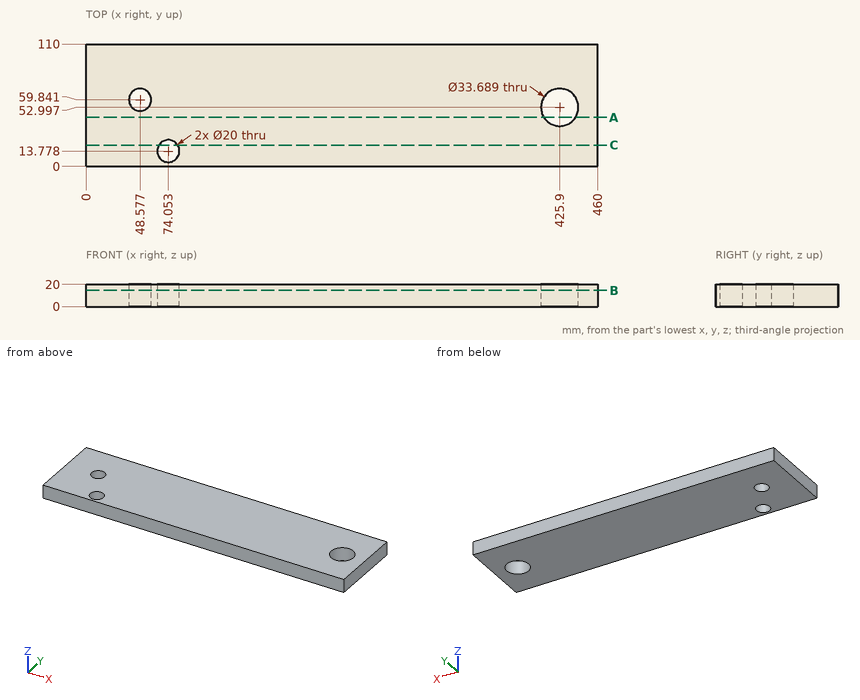
Design review of the part shown in the three views and the two pictorial views. Dimensions are in mm from the part's minimum x, y and z. Round coordinates to 2 decimals unless told otherwise and drop trailing zeros. Order: outer loops, then holes, each group sorted by start corner. A loop starts at its lowest first (then second) coordinate and runs counter-clockwise, first axis right, second up. Notation, with made-up numbers: (24, -4.5) -> (29, -4.5) arc R19 cw to (29, 24.5) -> close; hole circle Ø3 at (30.5, 6). An arc over 180 degrees is marked (long way). Write item = value, one per line. Start each with the question number.
1) Take a section at B-B on z = 14.5. State the section outline as (x, y) points (1 decimal).
2) Take a section at C-C on y = 19. State the section outline as (x, z) points (1 decimal), plus the area to 3 significant figures.
3) Take a section at A-A on y = 44. State the section outline as (x, z) points, plus the area to 3 significant figures.
4) Insertion check: pin 1 (20 mm diameter, centred on x = 425.9, y = 53, fed in from -Z). The pin has a flat end and moves straight along its axis. Give the tip position at first contact, or say it passes through.
5) To check wall thickness, follow line 1 (X direction, y = 15.5, z = 16.5) (1 decimal); line 2 (Y direction, x = 411.5, z = 13.75) (1 decimal); line 3 (X direction, y = 10.5, z = 9) (1 decimal). State the ranges of each line that lie inside material, in increasing order. Write a range as from..to.
Verdict:
q1.outline = (0, 0) -> (460, 0) -> (460, 110) -> (0, 110) -> close; hole circle Ø20 at (48.6, 59.8); hole circle Ø20 at (74.1, 13.8); hole circle Ø33.7 at (425.9, 53)
q2.outline = (0, 0) -> (65.5, 0) -> (65.5, 20) -> (0, 20) -> close; (82.6, 0) -> (460, 0) -> (460, 20) -> (82.6, 20) -> close
q2.area = 8,860 mm2
q3.outline = (0, 0) -> (411.66, 0) -> (411.66, 20) -> (0, 20) -> close; (440.14, 0) -> (460, 0) -> (460, 20) -> (440.14, 20) -> close
q3.area = 8,630 mm2
q4.pin_1 = through
q5.line_1 = 0..64.2, 83.9..460
q5.line_2 = 0..44.3, 61.7..110
q5.line_3 = 0..64.6, 83.5..460
